```python
from build123d import *

# Parameters (mm, degrees)
SKETCH1_W           = 20
SKETCH1_H           = 40.02889445
SKETCH1_H_2         = 40
SKETCH1_H_3         = 39.353713997
BOSS_EXTRUDE1_DEPTH = 4


with BuildPart() as part:
    # Sketch1 → Boss-Extrude1 (new body)
    with BuildSketch(Plane.XY):
        Polygon((66.836116993, 121.125108431), (-42.163883007, 121.125108431), (-42.163883007, 111.125108431), (-46.163883007, 111.125108431), (-46.163883007, 91.125108431), (-42.163883007, 91.125108431), (-42.163883007, 51.125108431), (-46.163883007, 51.125108431), (-46.163883007, 31.125108431), (-42.163883007, 31.125108431), (-42.163883007, -8.874891569), (-46.163883007, -8.874891569), (-46.163883007, -28.874891569), (-42.163883007, -28.874891569), (-42.163883007, -68.874891569), (-46.163883007, -68.874891569), (-46.163883007, -88.874891569), (-42.163883007, -88.874891569), (-42.163883007, -103.874891569), (66.836116993, -103.874891569), (66.836116993, -88.874891569), (70.836116993, -88.874891569), (70.836116993, -68.874891569), (66.836116993, -68.874891569), (66.836116993, -28.874891569), (70.836116993, -28.874891569), (70.836116993, -8.874891569), (66.836116993, -8.874891569), (66.836116993, 31.125108431), (70.836116993, 31.125108431), (70.836116993, 51.125108431), (66.836116993, 51.125108431), (66.836116993, 91.125108431), (70.836116993, 91.125108431), (70.836116993, 111.125108431), (66.836116993, 111.125108431), align=None)
        with Locations((43.223488174, -48.291018479)):
            Rectangle(SKETCH1_W, SKETCH1_H, mode=Mode.SUBTRACT)
        with Locations((-18.551254188, 82.990248393)):
            Rectangle(SKETCH1_W, SKETCH1_H_2, mode=Mode.SUBTRACT)
        with Locations((-18.551254188, 12.271619921)):
            Rectangle(SKETCH1_W, SKETCH1_H_3, mode=Mode.SUBTRACT)
        with Locations((-18.551254188, -48.291018479)):
            Rectangle(SKETCH1_W, SKETCH1_H, mode=Mode.SUBTRACT)
        with Locations((43.223488174, 12.271619921)):
            Rectangle(SKETCH1_W, SKETCH1_H_3, mode=Mode.SUBTRACT)
        with Locations((43.223488174, 82.990248393)):
            Rectangle(SKETCH1_W, SKETCH1_H_2, mode=Mode.SUBTRACT)
    extrude(amount=BOSS_EXTRUDE1_DEPTH)


solid = part.part
```
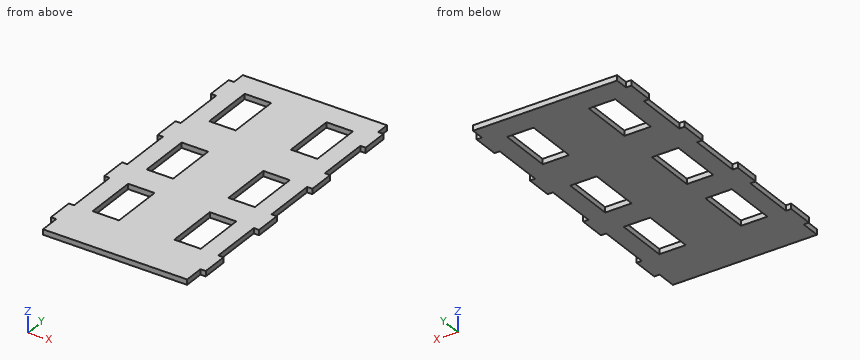
The model under review builds one solid part; all positions refer to its coordinate system, in mm. Round coordinates to 2 decimals unless told otherwise and drop trailing zeros. Loops run counter-clockwise (first coordinate to the right, second up) from the corner with the lowest first, then second, coordinate; pieces in that order, holes last. Notation, with made-up numbers: (80.5, -8.75) - (117.5, -8.75) arc R17 ccw to (117.5, 11.25) - close; hole circle Ø2 at (-37.5, 5). An arc over 180 degrees is marked (long way). Use a Markdown table: item, result. Add a question column.
Q1. Add section A-A (x = 37.5). State the section outline as (y, z) points, plus the area to 3 significant figures.
Q2. For probe 1 along X at (y, z) = (15.5, 2.9); probe 2 along Y at (x, z) = (-16.5, 3.85); probe 3 along X at (y, z) = (93.5, 2.95), list the stretches that pass through material, from the lowest coordinate up.
Q3. Add section C-C (z = 1.85). State how many separate pieces and enclosed holes the cut face has, plus the area to 3 significant figures.
Q4. Add section B-B (y = 68). State the section outline as (x, z) points, plus the area to 3 significant figures.
Q5. Insertion check: pin 1 Ø2 at (y, z) = (-95, 3) entering from +X; pin 2 Ø2 at (y, z) = (118, 2) entering from -X; pin 3 Ø10 at (x, y) = (-15, 89.5) entering from +Z; pin 4 Ø2 at (x, z) = (-44, 1.5) entering from -Y. Each pin has a flat end and moves straight along its axis. Give the tip position at first contact, or say it passes through.
Worked answers:
| question | item | result |
|---|---|---|
| 1 | outline | (-103.87, 0) - (-68.31, 0) - (-68.31, 4) - (-103.87, 4) - close; (-28.28, 0) - (-7.41, 0) - (-7.41, 4) - (-28.28, 4) - close; (31.95, 0) - (62.99, 0) - (62.99, 4) - (31.95, 4) - close; (102.99, 0) - (121.13, 0) - (121.13, 4) - (102.99, 4) - close |
| 1 | area | 422 mm² |
| 2 | probe 1 | -42.16 to -28.55, -8.55 to 33.22, 53.22 to 66.84 |
| 2 | probe 2 | -103.87 to -68.31, -28.28 to -7.41, 31.95 to 62.99, 102.99 to 121.13 |
| 2 | probe 3 | -46.16 to -28.55, -8.55 to 33.22, 53.22 to 70.84 |
| 3 | separate pieces | 1 |
| 3 | enclosed holes | 6 |
| 3 | area | 20,400 mm² |
| 4 | outline | (-42.16, 0) - (-28.55, 0) - (-28.55, 4) - (-42.16, 4) - close; (-8.55, 0) - (33.22, 0) - (33.22, 4) - (-8.55, 4) - close; (53.22, 0) - (66.84, 0) - (66.84, 4) - (53.22, 4) - close |
| 4 | area | 276 mm² |
| 5 | pin 1 | x = 66.84 |
| 5 | pin 2 | x = -42.16 |
| 5 | pin 3 | through |
| 5 | pin 4 | y = -88.87 |
